```python
from build123d import *

# Parameters (mm, degrees)
SKETCH_W        = 12.7
SKETCH_H        = 13.2
PAD_DEPTH       = 9.5
SKETCH004_W     = 10
SKETCH004_H     = 9.5
POCKET_DEPTH    = 0.5
POCKET001_DEPTH = 0.5


with BuildPart() as part:
    # Sketch → Pad (new body)
    with BuildSketch(Plane.XY):
        Rectangle(SKETCH_W, SKETCH_H)
    extrude(amount=PAD_DEPTH)

    # Sketch004 → Pocket (cut)
    with BuildSketch(Plane.YZ.offset(6.35)):
        with Locations((0, 4.75)):
            Rectangle(SKETCH004_W, SKETCH004_H)
    pocket = extrude(amount=-POCKET_DEPTH, mode=Mode.SUBTRACT)

    # Mirrored: Pocket across YZ
    add(pocket.mirror(Plane.YZ), mode=Mode.SUBTRACT)

    # Sketch005 → Pocket001 (cut)
    with BuildSketch(Plane.XY.offset(9.5)):
        Polygon((-6.35, 6.6), (6.35, 6.6), (6.35, 5), (5.85, 5), (5.85, 0), (-5.85, 0), (-5.85, 5), (-6.35, 5), align=None)
    pocket001 = extrude(amount=-POCKET001_DEPTH, mode=Mode.SUBTRACT)

    # Mirrored001: Pocket001 across XZ
    add(pocket001.mirror(Plane.XZ), mode=Mode.SUBTRACT)


solid = part.part
```
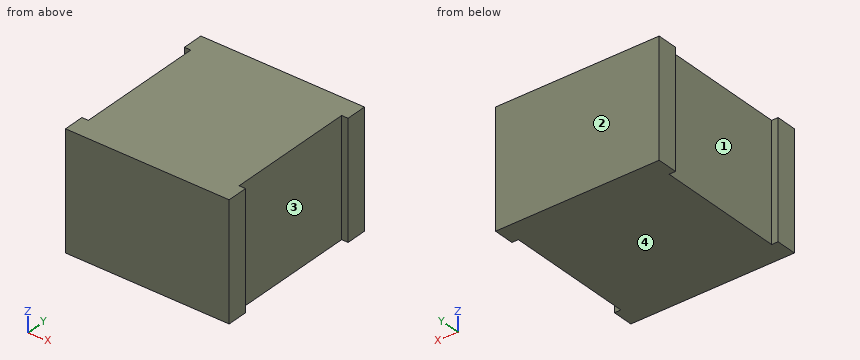
Work out the finished part from the listing and answer in its coordinate system (mm). Face numbers are marked on the shaded views. Coordinates: 2 decimals unless noted, no trailing zeros. Loops run counter-clockwise (first coordinate to the right, second up) from the corner with the lowest first, then second, coordinate; pieces in that order, holes last. Notation, with made-up numbers: (-3.5, 68) -> (18.5, 68) arc R18 ccw to (18.5, 74) -> close; hole circle Ø9 at (-26.5, 23). An arc over 180 degrees is marked (long way). Answer as CSV lines item,"result".
Q1. Each of these flat-tipped pins is pushed along its axis until it touches: pin 1 (4 mm diameter, centred on y = -1.5, z = 4.5, fed in from -X); pin 2 (4.5 mm diameter, centred on y = 1.5, z = 3.5, fed in from +X). Where does it stop, or does it pass through?
Findings:
pin 1,"stops at x = -5.85"
pin 2,"stops at x = 5.85"
Q2. Find the intervals of material crossed by probe 1 along X at (y, z) = (-4, 8.75), in increasing order.
Findings:
probe 1,"x = -5.85 to 5.85"
Q3. The part is cut by section A-A on z = 6. Write down the section's boundary in (x, y), and give its area (3 significant figures).
Findings:
outline,"(-6.35, -6.6) -> (6.35, -6.6) -> (6.35, -5) -> (5.85, -5) -> (5.85, 5) -> (6.35, 5) -> (6.35, 6.6) -> (-6.35, 6.6) -> (-6.35, 5) -> (-5.85, 5) -> (-5.85, -5) -> (-6.35, -5) -> close"
area,"158 mm²"
Q4. For a pull along Y with two mould halves and no side action, classify the marked faces 1, 2, 3 and 4 as +Y half, -Y half, draft (parallel to the pull), parting line (faces both ways), or undercut.
Findings:
face 1,"undercut"
face 2,"+Y half"
face 3,"undercut"
face 4,"draft"
Q5. The part is cut by section B-B on y = 0. Write down the section's boundary in (x, z), and give its area (3 significant figures).
Findings:
outline,"(-5.85, 0) -> (5.85, 0) -> (5.85, 9) -> (-5.85, 9) -> close"
area,"105 mm²"
